```python
from build123d import *

# Parameters (mm, degrees)
SKETCH1_R           = 1.25
SKETCH1_R_2         = 2
BOSS_EXTRUDE1_DEPTH = 5
SKETCH2_R           = 2.25
CUT_EXTRUDE1_DEPTH  = 1.5


with BuildPart() as part:
    # Sketch1 → Boss-Extrude1 (new body)
    with BuildSketch(Plane.XY):
        with BuildLine():
            Line((-32, -24.928932188), (-39.071067812, -32))
            ThreePointArc((-39.071067812, -32), (-39.071067812, -39.071067812), (-32, -39.071067812))
            Line((-32, -39.071067812), (-24.928932188, -32))
            Line((-24.928932188, -32), (24.928932188, -32))
            Line((24.928932188, -32), (32, -39.071067812))
            ThreePointArc((32, -39.071067812), (39.071067812, -39.071067812), (39.071067812, -32))
            Line((39.071067812, -32), (32, -24.928932188))
            Line((32, -24.928932188), (32, 24.928932188))
            Line((32, 24.928932188), (39.071067812, 32))
            ThreePointArc((39.071067812, 32), (39.071067812, 39.071067812), (32, 39.071067812))
            Line((32, 39.071067812), (24.928932188, 32))
            Line((24.928932188, 32), (-24.928932188, 32))
            Line((-24.928932188, 32), (-32, 39.071067812))
            ThreePointArc((-32, 39.071067812), (-39.071067812, 39.071067812), (-39.071067812, 32))
            Line((-39.071067812, 32), (-32, 24.928932188))
            Line((-32, 24.928932188), (-32, -24.928932188))
        make_face()
        with Locations((3.125, -5.412658774)):
            Circle(SKETCH1_R, mode=Mode.SUBTRACT)
        with Locations((-6.25, 0)):
            Circle(SKETCH1_R, mode=Mode.SUBTRACT)
        with Locations((3.125, 5.412658774)):
            Circle(SKETCH1_R, mode=Mode.SUBTRACT)
        with Locations((-35.535533906, -35.535533906)):
            Circle(SKETCH1_R_2, mode=Mode.SUBTRACT)
        with Locations((35.535533906, -35.535533906)):
            Circle(SKETCH1_R_2, mode=Mode.SUBTRACT)
        with Locations((35.535533906, 35.535533906)):
            Circle(SKETCH1_R_2, mode=Mode.SUBTRACT)
        with Locations((-35.535533906, 35.535533906)):
            Circle(SKETCH1_R_2, mode=Mode.SUBTRACT)
    extrude(amount=BOSS_EXTRUDE1_DEPTH)

    # Sketch2 → Cut-Extrude1 (cut)
    with BuildSketch(Plane(origin=(0, 0, 0), x_dir=(-1, 0, 0), z_dir=(0, 0, -1))):
        with Locations((-3.125, 5.412658774)):
            Circle(SKETCH2_R)
        with Locations((-3.125, -5.412658774)):
            Circle(SKETCH2_R)
        with Locations((6.25, 0)):
            Circle(SKETCH2_R)
    extrude(amount=-CUT_EXTRUDE1_DEPTH, mode=Mode.SUBTRACT)


solid = part.part
```
CAD build for the part. Positions are in the model's coordinates, mm. A direction names the side the tool comes from. Round coordinates to 2 decimals unless told otherwise and drop trailing zeros. Order: outer loops, then holes, each group sorted by start corner. A loop starts at its lowest first (then second) coordinate and runs counter-clockwise, first axis right, second up. Notation, with made-up numbers: (12, 52) - (38, 52) arc R33 cw to (38, 83) - close; hole circle Ø7 at (-27.5, 80.25). An arc over 180 degrees is marked (long way). Use CSV: the item, a comma, the result in double quotes. Start each with the question number.
1) Saw through at C-C (z = 3.1). List the corners of the cut face in (x, y) (3 decimals), and give its area (3 significant figures).
2) Saw through at D-D (x = -20). List the corners of the cut face in (y, z).
3) Saw through at A-A (y = 0). List the corners of the cut face in (x, z).
4) Pin check, flat tips, straight feed: pin 1 Ø3.5 at (x, y) = (3.12, -5.41) entering from -Z; pin 2 Ø2.5 at (x, z) = (11.5, 1.5) entering from +Y; pin 3 Ø2 at (y, z) = (-7, 3) entering from +X. Stop position of each tip, or through.
5) Saw through at B-B (x = -6.25). List the corners of the cut face in (y, z), and give its area (4 significant figures).
6) Two-plate mould, pull along Y, no slides. Class faces 4 (the flat face through (-35.585, 28.514, 2.465)), 5 (the flat face through (-1, 1, 0)), 6 (the flat face through (0, 32, 2)): pulls with the +Y half, pulls with the -Y half, needs draft (parallel to the pull), parting line crosses it, or undercut.
7) Wall check: L1, parallel to Y at x = -35, z = 1; L2, parallel to X at y = -7.5, z = 2.8. Give the ranges that are in metal, low to high. Write a range as [from, to].
8) Tool access for faces 1 (the flat face through (2, 4, 1.5)), 2 (the flat face through (-32, 0, 2)), 3 (the flat face through (35.486, 28.415, 2.465)): list every direction of +Z, -Z, +X, -X, +Y, -Y with a clear straight run to the whole face (end or side of a thin tool).
Values follow:
1,outline,"(-39.071, -32) arc R5 ccw to (-32, -39.071) - (-24.929, -32) - (24.929, -32) - (32, -39.071) arc R5 ccw to (39.071, -32) - (32, -24.929) - (32, 24.929) - (39.071, 32) arc R5 ccw to (32, 39.071) - (24.929, 32) - (-24.929, 32) - (-32, 39.071) arc R5 ccw to (-39.071, 32) - (-32, 24.929) - (-32, -24.929) - close; hole circle Ø4 at (-35.536, -35.536); hole circle Ø4 at (-35.536, 35.536); hole circle Ø2.5 at (-6.25, 0); hole circle Ø2.5 at (3.125, -5.413); hole circle Ø2.5 at (3.125, 5.413); hole circle Ø4 at (35.536, -35.536); hole circle Ø4 at (35.536, 35.536)"
1,area,"4,490 mm2"
2,outline,"(-32, 0) - (32, 0) - (32, 5) - (-32, 5) - close"
3,outline,"(-32, 0) - (-8.5, 0) - (-8.5, 1.5) - (-7.5, 1.5) - (-7.5, 5) - (-32, 5) - close; (-5, 1.5) - (-4, 1.5) - (-4, 0) - (32, 0) - (32, 5) - (-5, 5) - close"
4,pin 1,"stops at z = 1.5"
4,pin 2,"stops at y = 32"
4,pin 3,"stops at x = 32"
5,outline,"(-32, 0) - (-2.25, 0) - (-2.25, 1.5) - (-1.25, 1.5) - (-1.25, 5) - (-32, 5) - close; (1.25, 1.5) - (2.25, 1.5) - (2.25, 0) - (32, 0) - (32, 5) - (1.25, 5) - close"
5,area,"304.5 mm2"
6,face 4,"undercut"
6,face 5,"needs draft"
6,face 6,"pulls with the +Y half"
7,L1,"y = [-40.51, -37.46], [-33.61, -27.93], [27.93, 33.61], [37.46, 40.51]"
7,L2,"x = [-32, 32]"
8,face 1,"-Z"
8,face 2,"+Z, -Z, -X"
8,face 3,"+Z, -Z, +X"
